Could you check a few things on this model? Use its own coordinates, in mm. Face numbers are marked on the shaded views. A direction names the side the tool comes from. Coordinates: 2 decimals unless noted, no trailing zeros. Order: outer loops, then holes, each group sorted by start corner. A loop starts at its lowest first (then second) coordinate and runs counter-clockwise, first axis right, second up. Notation, with made-up numbers: M 0.5,83.25 L 13.5,83.25 A28 cw 13.5,120.25 Z; hole C -23,-21 d1. An arc over 180 degrees is marked long. Put each result on its own line as item: value. Start each with the question number.
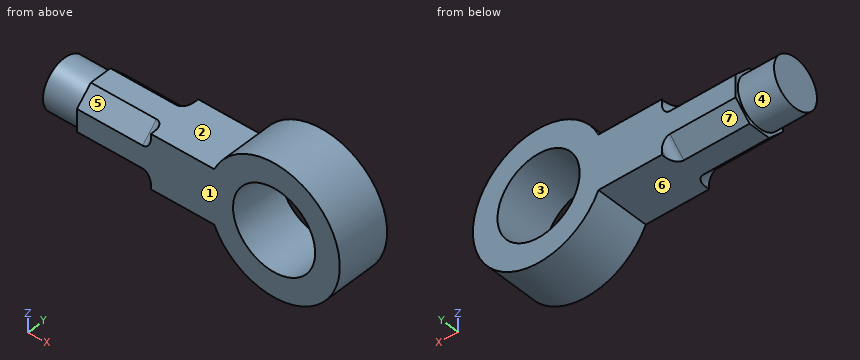
```python
from build123d import *

# Parameters (mm, degrees)
SKETCH1_R                = 40
SKETCH1_R_2              = 25
BOSS_EXTRUDE1_DEPTH      = 18
BOSS_EXTRUDE2_DEPTH      = 45
SKETCH3_R                = 15
BOSS_EXTRUDE3_DEPTH      = 22
BOSS_EXTRUDE4_REACH      = 125.081
SKETCH4_W                = 33
SKETCH4_H                = 33
FILLET1_R                = 5
FILLET7_R                = 1.5
SCALA2_SCALE             = 0.1
SCHIZZO3_W               = 13.390862708
SCHIZZO3_H               = 12.193146248
TAGLIO_ESTRUSIONE3_DEPTH = 0.15
SCHIZZO4_W               = 17.573052966
SCHIZZO4_H               = 12.055703376
TAGLIO_ESTRUSIONE4_DEPTH = 0.15


with BuildPart() as part:
    # Sketch1 → Boss-Extrude1 (new, symmetric)
    with BuildSketch(Plane(origin=(0, 0, 0), x_dir=(1, 0, 0), z_dir=(0, 1, 0))):
        with Locations(Location((0, 0, 0), (0, 0, 270))):
            Circle(SKETCH1_R)
        with Locations(Location((0, 0, 0), (0, 0, 270))):
            Circle(SKETCH1_R_2, mode=Mode.SUBTRACT)
    extrude(amount=BOSS_EXTRUDE1_DEPTH, both=True)

    # Sketch4 → Boss-Extrude4 (add, up to next)
    with BuildSketch(Plane(origin=(-75, 0, 0), x_dir=(0, 0, -1), z_dir=(1, 0, 0)), mode=Mode.PRIVATE) as boss_extrude4_sk1:
        Rectangle(SKETCH4_W, SKETCH4_H)
    boss_extrude4_tool1 = extrude(boss_extrude4_sk1.sketch, amount=BOSS_EXTRUDE4_REACH, mode=Mode.PRIVATE) - part.part


with BuildPart() as body_2:
    # Sketch2 → Boss-Extrude2 (new body)
    with BuildSketch(Plane(origin=(-120, 0, 0), x_dir=(0, 0, -1), z_dir=(1, 0, 0))):
        Polygon((-16.5, 6.834523779), (-16.5, -6.834523779), (-6.834523779, -16.5), (6.834523779, -16.5), (16.5, -6.834523779), (16.5, 6.834523779), (6.834523779, 16.5), (-6.834523779, 16.5), align=None)
    extrude(amount=BOSS_EXTRUDE2_DEPTH)

    # Sketch3 → Boss-Extrude3 (add)
    with BuildSketch(Plane(origin=(-120, 0, 0), x_dir=(0, 0, -1), z_dir=(1, 0, 0))):
        Circle(SKETCH3_R)
    extrude(amount=-BOSS_EXTRUDE3_DEPTH)


with BuildPart() as part_1:
    add(part.part)

    add(body_2.part)  # Boss-Extrude4 merges body 2
    add(boss_extrude4_tool1.solids().sort_by_distance((-75, 0, 0))[0])

    # Fillet1
    fillet1_edges = [part_1.edges().sort_by_distance(p)[0] for p in [
        (-75, 11.66726189, 11.66726189),
        (-75, -11.66726189, 11.66726189),
        (-75, -11.66726189, -11.66726189),
        (-75, 11.66726189, -11.66726189),
    ]]
    fillet(fillet1_edges, radius=FILLET1_R)

    # Fillet7
    fillet7_edges = [part_1.edges().sort_by_distance(p)[0] for p in [
        (-40, -16.5, 0),
        (-40, 16.5, 0),
    ]]
    fillet(fillet7_edges, radius=FILLET7_R - 0.0001)  # a hair under: the kernel refuses the full size


with BuildPart() as part_2:
    # Scala2: scaled about (-40.064009794, 0, -1e-09)
    add(part_1.part.scale(SCALA2_SCALE).moved(Location((-36.057608815, 0, -1e-09))))

    # Schizzo3 → Taglio-Estrusione3 (cut)
    with BuildSketch(Plane(origin=(0, 1.8, 0), x_dir=(1, 0, 0), z_dir=(0, 1, 0))):
        with Locations((-35.542120141, -0.94246541)):
            Rectangle(SCHIZZO3_W, SCHIZZO3_H)
    extrude(amount=-TAGLIO_ESTRUSIONE3_DEPTH, mode=Mode.SUBTRACT)

    # Schizzo4 → Taglio-Estrusione4 (cut)
    with BuildSketch(Plane.XZ.offset(1.8)):
        with Locations((-38.634584769, -0.834474582)):
            Rectangle(SCHIZZO4_W, SCHIZZO4_H)
    extrude(amount=-TAGLIO_ESTRUSIONE4_DEPTH, mode=Mode.SUBTRACT)


solid = part_2.part
```
Item 1: I need wall thicknesses on probe 1 along X at (y, z) = (-0.7, 0); probe 2 along Z at (x, y) = (-44.75, -0.1); probe 3 along Z at (x, y) = (-36.5, -0.6). Which ranges of each line are inside material? Lowest first, please.
Item 2: If we section it at A-A on z = 0: Write out the boundary of the cut face in (x, y), then the cut area to 3 significant figures.
Item 3: If we section it at D-D on y = 0: Write out the boundary of the cut face in (x, z), then the cut area to 3 significant figures.
Item 4: If we section it at B-B on x = -35: Write out the boundary of the cut face in (y, z).
Item 5: For the marked faces 4, 5, 6 and 7, which set-ups out of +Z, -Z, +X, -X, +Y, -Y let a thin tool reach every point of the face, with its end or its side?
Item 6: If we mould it in two halves opening along Z, with no side actions, what happens to the marked faces 1, 2 and 3? For each: released by +Z, released by -Z, zero draft, split by the parting line, or undercut.
Item 7: If we section it at C-C on x = -46.5: Write out the boundary of the cut face in (y, z).
Geometry check:
1. probe 1: x = -50.26 to -38.56, -33.56 to -32.06
1. probe 2: z = -1.65 to 1.65
1. probe 3: z = -3.98 to -2.46, 2.46 to 3.98
2. outline: M -50.26,-1.5 L -48.06,-1.5 L -48.06,-1.65 L -38.56,-1.65 L -38.56,1.65 L -48.06,1.65 L -48.06,1.5 L -50.26,1.5 Z; M -33.56,-1.65 L -32.06,-1.65 L -32.06,1.65 L -33.56,1.65 Z
2. area: 42.9 mm²
3. outline: M -50.26,-1.5 L -48.06,-1.5 L -48.06,-1.65 L -39.7,-1.65 A4 ccw long -39.7,1.65 L -48.06,1.65 L -48.06,1.5 L -50.26,1.5 Z; hole C -36.06,0 d5
3. area: 64.0 mm²
4. outline: M -1.65,-3.86 L 1.65,-3.86 L 1.65,-2.27 L -1.65,-2.27 Z; M -1.65,2.27 L 1.65,2.27 L 1.65,3.86 L -1.65,3.86 Z
5. face 4: -X
5. face 5: +Z, -X, -Y
5. face 6: -Z, -X, +Y, -Y
5. face 7: -Z, -X, +Y
6. face 1: zero draft
6. face 2: released by +Z
6. face 3: undercut
7. outline: M -1.65,-0.68 L -0.68,-1.65 L 0.68,-1.65 L 1.65,-0.68 L 1.65,0.68 L 0.68,1.65 L -0.68,1.65 L -1.65,0.68 Z
